```python
from build123d import *

# Parameters (mm, degrees)
F0_R     = 5
F1_DEPTH = 80
F3_R     = 7.5
F4_DEPTH = 36
F6_DEPTH = 14


with BuildPart() as f1:
    # F0 (on Right) → F1 (new body)
    with BuildSketch(Plane.YZ):
        Circle(F0_R)
    extrude(amount=F1_DEPTH)

    # F3 (on offset) → F4 (join)
    with BuildSketch(Plane.YZ.offset(14)):
        Circle(F3_R)
    extrude(amount=F4_DEPTH)

    # F5 (on face) → F6 (cut, through all)
    with BuildSketch(Plane(origin=(0, 0, 0), x_dir=(0, -1, 0), z_dir=(-1, 0, 0))):
        with BuildLine():
            Line((-4, -3), (-4, 3))
            ThreePointArc((-4, 3), (-5, 0), (-4, -3))
        make_face()
        with BuildLine():
            ThreePointArc((4, -3), (5, 0), (4, 3))
            Line((4, 3), (4, -3))
        make_face()
    extrude(amount=-F6_DEPTH, mode=Mode.SUBTRACT)


solid = f1.part
```
Source: CAD feature listing. Evaluate the final solid. Frame: model axes, mm. A direction names the side the tool comes from. Round coordinates to 2 decimals unless told otherwise and drop trailing zeros. Order: outer loops, then holes, each group sorted by start corner. A loop starts at its lowest first (then second) coordinate and runs counter-clockwise, first axis right, second up. Notation, with made-up numbers: (-37, 5.25) -> (9, 5.25) arc R5 cw to (9, 14.25) -> close; hole circle Ø9 at (-36, 40). An arc over 180 degrees is marked (long way). Use CSV: the item, a comma, the result in double quotes.
(1) Section A-A on z = 0. Return the cut outline in (x, y).
Report:
outline,"(0, -4) -> (14, -4) -> (14, -7.5) -> (50, -7.5) -> (50, -5) -> (80, -5) -> (80, 5) -> (50, 5) -> (50, 7.5) -> (14, 7.5) -> (14, 4) -> (0, 4) -> close"
(2) First-contact query: pin 1 Ø6.5 at (x, z) = (8, 1) entering from -Y; pin 2 Ø4 at (x, z) = (69, -2.5) entering from -Y; pin 3 Ø4 at (x, z) = (38.5, -3.5) entering from -Y. Flat tips, straight axial feed; report the tip coordinate or a pass-through.
Report:
pin 1,"y = -4"
pin 2,"y = -4.97"
pin 3,"y = -7.35"
(3) Access query for faces 1 (the face through (50, 2, -5)), 2 (the face through (7, -4, 0)), 3 (the face through (14, 5, 0)), 4 (the face through (7, 0, -5)), 5 (the face through (7, 4, 0)). Directions: +Z, -Z, +X, -X, +Y, -Y. A direction counts if a zero-diameter tool reaches every point of the face in a straight line with its end or side. Return the directions, or none.
Report:
face 1,"+X"
face 2,"+Z, -Z, -X, -Y"
face 3,"-X"
face 4,"-Z, -X"
face 5,"+Z, -Z, -X, +Y"
(4) Section C-C on x = 38. Return the cut outline in (y, z), and give its area (3 significant figures).
Report:
outline,"circle Ø15 at (0, 0)"
area,"177 mm^2"
(5) Ray query, L1, parallel to Y at x = 39, z = -0.5; L2, parallel to X at y = 4.75, z = 0; L3, parallel to X at y = 3, z = 5.5. Return the intervals inside material, ascending.
Report:
L1,"-7.48 to 7.48"
L2,"14 to 80"
L3,"14 to 50"
(6) Section B-B on y = 0. Return the cut outline in (x, z), and give its area (3 significant figures).
Report:
outline,"(0, -5) -> (14, -5) -> (14, -7.5) -> (50, -7.5) -> (50, -5) -> (80, -5) -> (80, 5) -> (50, 5) -> (50, 7.5) -> (14, 7.5) -> (14, 5) -> (0, 5) -> close"
area,"980 mm^2"
(7) Section D-D on z = 6.25. Return the cut outline in (x, y).
Report:
outline,"(14, -4.15) -> (50, -4.15) -> (50, 4.15) -> (14, 4.15) -> close"
